Geometry check sheet. Reference: the model listing, model coordinates, mm. Give positions to 0.01 mm unless a question says otherwise; leave off trailing zeros. Order: outer loops, then holes, each group sorted by start corner. A loop starts at its lowest first (then second) coordinate and runs counter-clockwise, first axis right, second up.
Autodesk Fusion 360 part; units mm, degrees
sketch "Sketch1" plane through (0, 0, 0) normal (0, 0, 1) x (1, 0, 0) in component "Laptop side"
  line L0 (0, 0) -> (225.9, 0)
  line L1 (225.9, 0) -> (225.9, 18.5)
  line L2 (225.9, 18.5) -> (0, 18.5)
  line L3 (0, 18.5) -> (0, 0)
  dimension "d1" = 225.9
  dimension "d2" = 18.5
extrude "Extrude1" add sketch "Sketch1" along normal blind 13.24 in component "Laptop side"
sketch "Sketch2" plane through (0, 0, 0) normal (0, -1, 0) x (1, 0, 0) in component "Laptop side"
  line L0 (0, 0) -> (225.9, 0)
  line L1 (225.9, 0) -> (225.9, 13.24)
  line L2 (225.9, 13.24) -> (0, 13.24)
  line L3 (0, 13.24) -> (0, 0)
  line L4 (16.56, 9.86) -> (23.66, 9.86)
  line L5 (23.66, 9.86) -> (23.66, 6.76)
  line L6 (23.66, 6.76) -> (16.56, 6.76)
  line L7 (16.56, 6.76) -> (16.56, 9.86)
  line L8 (33.96, 9.82) -> (40.16, 9.82)
  line L9 (41.56, 8.42) -> (41.56, 8.04)
  line L10 (40.16, 6.64) -> (33.96, 6.64)
  line L11 (32.56, 8.04) -> (32.56, 8.42)
  arc A0 (33.96, 9.82) -> (32.56, 8.42) centre (33.96, 8.42) ccw
  arc A1 (32.56, 8.04) -> (33.96, 6.64) centre (33.96, 8.04) ccw
  arc A2 (40.16, 6.64) -> (41.56, 8.04) centre (40.16, 8.04) ccw
  arc A3 (41.56, 8.42) -> (40.16, 9.82) centre (40.16, 8.42) ccw
  line L12 (49.66, 9.04) -> (72.76, 9.04)
  line L13 (73.46, 8.34) -> (73.46, 7.34)
  line L14 (72.76, 6.64) -> (49.66, 6.64)
  line L15 (48.96, 7.34) -> (48.96, 8.34)
  arc A4 (49.66, 9.04) -> (48.96, 8.34) centre (49.66, 8.34) ccw
  arc A5 (48.96, 7.34) -> (49.66, 6.64) centre (49.66, 7.34) ccw
  arc A6 (72.76, 6.64) -> (73.46, 7.34) centre (72.76, 7.34) ccw
  arc A7 (73.46, 8.34) -> (72.76, 9.04) centre (72.76, 8.34) ccw
  point P0 (32.56, 9.82)
  point P1 (41.56, 9.82)
  point P2 (32.56, 6.64)
  point P3 (48.96, 9.04)
  point P4 (73.46, 9.04)
  point P5 (48.96, 6.64)
  dimension "d5" = 7.1
  dimension "d6" = 3.1
  dimension "d7" = 16.56
  dimension "d8" = 3.38
  dimension "d19" = 9
  dimension "d20" = 3.18
  dimension "d21" = 1.4
  dimension "d22" = 3.42
  dimension "d24" = 25
  dimension "d25" = 8.9
  dimension "d26" = 24.5
  dimension "d27" = 2.4
  dimension "d28" = 4.2
  dimension "d29" = 56.9
  dimension "d30" = 25.3
  dimension "d31" = 0.7
extrude "Extrude2" cut sketch "Sketch2" against normal blind 9.5 contours L4 L5 L6 L7 | L8 L9 L10 L11 A0 A1 A2 A3 | L12 L13 L14 L15 A4 A5 A6 A7 in component "Laptop side"
fillet "Fillet1" radius 12 1 edges at (225.9, 0, 6.62) in component "Laptop side"
fillet "Fillet1" radius 11 1 edges at (0, 0, 6.62) in component "Laptop side"
component "Laptop side" placed x (1, 0, 0) y (0, 1, 0) z (0, 0, 1) at (0, 0, 0)
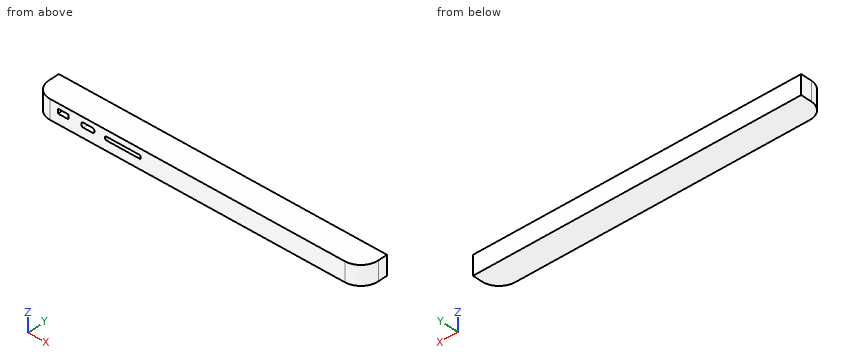
Item 1: Sectioned sample at B-B (x = 57). Enter the section's corners in (y, z), and give its area (3 significant figures).
Reported:
outline: (0, 0) - (18.5, 0) - (18.5, 13.24) - (0, 13.24) - (0, 9.04) - (9.5, 9.04) - (9.5, 6.64) - (0, 6.64) - close
area: 222 mm2
Item 2: Sectioned sample at A-A (y = 7.25). Enter the section's corners in (x, z).
Reported:
outline: (0.66, 0) - (224.92, 0) - (224.92, 13.24) - (0.66, 13.24) - close; hole (16.56, 6.76) - (23.66, 6.76) - (23.66, 9.86) - (16.56, 9.86) - close; hole (32.56, 8.04) arc R1.4 ccw to (33.96, 6.64) - (40.16, 6.64) arc R1.4 ccw to (41.56, 8.04) - (41.56, 8.42) arc R1.4 ccw to (40.16, 9.82) - (33.96, 9.82) arc R1.4 ccw to (32.56, 8.42) - close; hole (48.96, 7.34) arc R0.7 ccw to (49.66, 6.64) - (72.76, 6.64) arc R0.7 ccw to (73.46, 7.34) - (73.46, 8.34) arc R0.7 ccw to (72.76, 9.04) - (49.66, 9.04) arc R0.7 ccw to (48.96, 8.34) - close
Item 3: Gauge pin test, flat ends, axial feed: pin 1 (3.5 mm diameter, centred on y = 3.5, z = 8.5, fed in from -X); pin 2 (2.5 mm diameter, centred on x = 37.5, z = 9, fed in from -Y); pin 3 (1 mm diameter, centred on y = 11, z = 2.5, fed in from +X); pin 4 (0.8 mm diameter, centred on y = 6.5, z = 8, fed in from -X). Record the tip position at first contact, or that the pin passes through.
Reported:
pin 1: stops at x = 1.62
pin 2: stops at y = 0
pin 3: stops at x = 225.89
pin 4: stops at x = 0.79
Item 4: Scan lines: L1, parallel to Z at x = 70, y = 4; L2, parallel to X at y = 11, z = 4; L3, parallel to X at y = 6.5, z = 1.75. Record each from-to range of solid material in increasing order.
Reported:
L1: z = 0 to 6.64, 9.04 to 13.24
L2: x = 0 to 225.86
L3: x = 0.96 to 224.57
